The listing builds one solid part. Answer for the finished solid, in the listing's coordinates (mm). A direction names the side the tool comes from. Give positions to 0.01 mm unless a question says otherwise; leave off trailing zeros. Loops run counter-clockwise (first coordinate to the right, second up) from the corner with the lowest first, then second, coordinate; pieces in that order, holes last. Notation, with made-up numbers: (-39, 43) - (-20, 43) arc R16 ccw to (-20, 54) - close; hole circle Ø5 at (-28.75, 18.25). An arc over 180 degrees is marked (long way). Answer in a Markdown table with one row per item. Add a question column.
```python
from build123d import *

# Parameters (mm, degrees)
F0_W     = 70
F0_H     = 70
F1_DEPTH = 130
F2_T     = -2.5
F3_W     = 60
F3_H     = 60
F4_DEPTH = 25
F5_W     = 10
F5_H     = 10
F6_DEPTH = 25


with BuildPart() as f1:
    # F0 (on Front) → F1 (new body)
    with BuildSketch(Plane.XZ):
        with Locations((-6.760671, 9.284316)):
            Rectangle(F0_W, F0_H)
    extrude(amount=F1_DEPTH)

    # F2
    f2_openings = [f1.faces().sort_by_distance(p)[0] for p in [
        (-6.760671, -65, 44.284316),
    ]]
    offset(amount=F2_T, openings=f2_openings)

    # F3 (on Front) → F4 (cut)
    with BuildSketch(Plane.XZ):
        with Locations((-6.760671, 9.284316)):
            Rectangle(F3_W, F3_H)
    extrude(amount=F4_DEPTH, mode=Mode.SUBTRACT)

    # F5 (on face) → F6 (cut)
    with BuildSketch(Plane.XY.offset(-23.215684)):
        with Locations((-6.760671, -77.5)):
            Rectangle(F5_W, F5_H)
    extrude(amount=-F6_DEPTH, mode=Mode.SUBTRACT)


solid = f1.part
```
(1) A cutting plane is placed at B-B on y = -81. Determine the outline of the cut face in (x, z), plus the area to 4 significant figures.
(2) A cutting plane is placed at C-C on z = 14.5. Determine the outline of the cut face in (x, y).
(3) A tool of negligible diameter and unlimited length cuts with its end or side. For faces 1 (the face through (-7, -130, 10)), 2 (the face through (-7, -82.5, -24)), 3 (the face through (-39.261, -64, 10)), 4 (the face through (28.239, -64, 9)), 5 (the face through (-7, -1, -20.716)), from which of +Z, -Z, +X, -X, +Y, -Y can it reach the whole face along a straight path? Write none if from no direction.
(4) A cutting plane is placed at A-A on x = 18. Determine the outline of the cut face in (y, z), plus the area to 4 significant figures.
(5) Given pin 1 Ø4 at (x, y) = (-22.5, -55.5) entering from +Z; pin 2 Ø10 at (x, z) = (-20.5, 22.5) entering from +Y, each flat-ended and moving along its own axis, determine where each tip first touches the part or whether it passes through.
(6) The mould has two halves that part along X. Classify faces 6 (the face through (25.739, -64, 10)), 7 (the face through (-41.761, -64, 9)), 8 (the face through (-36.761, -1, 9)), 9 (the face through (-38, 0, 10)): pulls with the +X half, pulls with the -X half, needs draft (parallel to the pull), parting line crosses it, or undercut.
(7) Find the intervals of material crossed by line 1 along X through (y, z) = (-93, -18.5); line 2 along Y through (x, z) = (25.5, 14); line 3 along Y through (x, z) = (-30.5, 24.5), in increasing order. Write a range as [from, to].
(8) A cutting plane is placed at D-D on y = -96.5. Determine the outline of the cut face in (x, z), plus the area to 4 significant figures.
Evaluation:
| question | item | result |
|---|---|---|
| 1 | outline | (-41.76, -25.72) - (-11.76, -25.72) - (-11.76, -23.22) - (-39.26, -23.22) - (-39.26, 44.28) - (-41.76, 44.28) - close; (-1.76, -25.72) - (28.24, -25.72) - (28.24, 44.28) - (25.74, 44.28) - (25.74, -23.22) - (-1.76, -23.22) - close |
| 1 | area | 487.5 mm² |
| 2 | outline | (-41.76, -130) - (28.24, -130) - (28.24, 0) - (23.24, 0) - (23.24, -2.5) - (25.74, -2.5) - (25.74, -127.5) - (-39.26, -127.5) - (-39.26, -2.5) - (-36.76, -2.5) - (-36.76, 0) - (-41.76, 0) - close |
| 3 | face 1 | +Z, -Z, +X, -X, -Y |
| 3 | face 2 | +Z, -Z |
| 3 | face 3 | +Z |
| 3 | face 4 | +Z, -Z, +X, +Y, -Y |
| 3 | face 5 | +Y |
| 4 | outline | (-130, -25.72) - (0, -25.72) - (0, -20.72) - (-2.5, -20.72) - (-2.5, -23.22) - (-127.5, -23.22) - (-127.5, 44.28) - (-130, 44.28) - close; (-2.5, 39.28) - (0, 39.28) - (0, 44.28) - (-2.5, 44.28) - close |
| 4 | area | 512.5 mm² |
| 5 | pin 1 | stops at z = -23.22 |
| 5 | pin 2 | stops at y = -127.5 |
| 6 | face 6 | undercut |
| 6 | face 7 | pulls with the -X half |
| 6 | face 8 | undercut |
| 6 | face 9 | needs draft |
| 7 | line 1 | x = [-41.76, -39.26], [25.74, 28.24] |
| 7 | line 2 | y = [-130, -127.5], [-2.5, 0] |
| 7 | line 3 | y = [-130, -127.5] |
| 8 | outline | (-41.76, -25.72) - (28.24, -25.72) - (28.24, 44.28) - (25.74, 44.28) - (25.74, -23.22) - (-39.26, -23.22) - (-39.26, 44.28) - (-41.76, 44.28) - close |
| 8 | area | 512.5 mm² |
